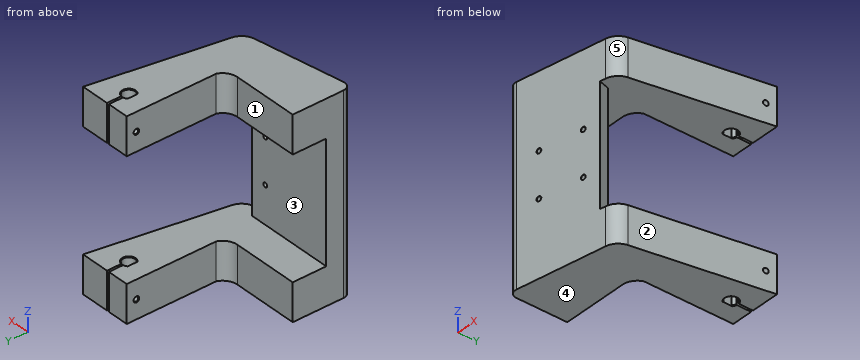
from build123d import *

# Parameters (mm, degrees)
BOSS_EXTRUDE1_DEPTH = 65
CUT_EXTRUDE1_DEPTH  = 40
CUT_EXTRUDE4_DEPTH  = 22.5
SKETCH11_W          = 20
SKETCH11_H          = 25
BOSS_EXTRUDE2_DEPTH = 10
BOSS_EXTRUDE6_DEPTH = 25
BOSS_EXTRUDE7_DEPTH = 25
CUT_EXTRUDE16_DEPTH = 130
SKETCH27_R          = 1.5
CUT_EXTRUDE17_DEPTH = 50
SKETCH28_R          = 1.7
CUT_EXTRUDE18_DEPTH = 50
BOSS_EXTRUDE8_DEPTH = 25
BOSS_EXTRUDE9_DEPTH = 25
CHAMFER9_SIZE       = 0.4
SKETCH31_R          = 1.5
CUT_EXTRUDE19_DEPTH = 10
FILLET1_R           = 0.2


with BuildPart() as part:
    # Sketch1 → Boss-Extrude1 (new body, symmetric)
    with BuildSketch(Plane.XY):
        with BuildLine():
            Line((0, 0), (0, -25.554938316))
            ThreePointArc((0, -25.554938316), (-2.359933303, -32.007021768), (-8.325876175, -35.413807897))
            Line((-8.325876175, -35.413807897), (-67.775097409, -45.508814922))
            ThreePointArc((-67.775097409, -45.508814922), (-71.838201048, -44.399413479), (-73.612159322, -40.579380131))
            Line((-73.612159322, -40.579380131), (-73.612159322, -6.5))
            Line((-73.612159322, -6.5), (-29.367881905, -6.5))
            ThreePointArc((-29.367881905, -6.5), (-23.632117541, -4.691520443), (-19.970955697, 0.079798567))
            Line((-19.970955697, 0.079798567), (-20, 0))
            Line((-20, 0), (0, 0))
        make_face()
    extrude(amount=BOSS_EXTRUDE1_DEPTH, both=True)

    # Sketch2 → Cut-Extrude1 (cut, symmetric)
    with BuildSketch(Plane.XY):
        with BuildLine():
            Line((-20, 0), (-19.970955697, 0.079798567))
            ThreePointArc((-19.970955697, 0.079798567), (-20.672372291, -1.438432196), (-21.617003148, -2.818534521))
            Line((-21.617003148, -2.818534521), (-12.102051753, -36.055036129))
            Line((-12.102051753, -36.055036129), (-8.325876175, -35.413807897))
            ThreePointArc((-8.325876175, -35.413807897), (-2.359933303, -32.007021768), (0, -25.554938316))
            Line((0, -25.554938316), (0, 0))
            Line((0, 0), (-20, 0))
        make_face()
    extrude(amount=CUT_EXTRUDE1_DEPTH, both=True, mode=Mode.SUBTRACT)

    # Sketch5 → Cut-Extrude4 (cut, symmetric)
    with BuildSketch(Plane(origin=(0, -6.5, 0), x_dir=(1, 0, 0), z_dir=(0, 1, 0))):
        Polygon((-73.612159322, 40), (-29.401702386, 40), (0, 40), (0, -40), (-29.367881905, -40), (-73.612159322, -40), align=None)
    extrude(amount=CUT_EXTRUDE4_DEPTH, both=True, mode=Mode.SUBTRACT)

    # Sketch11 → Boss-Extrude2 (add)
    with BuildSketch(Plane(origin=(0, 0, 0), x_dir=(1, 0, 0), z_dir=(0, 1, 0))):
        with Locations((-10, 52.5)):
            Rectangle(SKETCH11_W, SKETCH11_H)
        with Locations((-10, -52.5)):
            Rectangle(SKETCH11_W, SKETCH11_H)
    extrude(amount=BOSS_EXTRUDE2_DEPTH)

    # Sketch24 → Boss-Extrude6 (add)
    with BuildSketch(Plane(origin=(0, 0, -65), x_dir=(-1, 0, 0), z_dir=(0, 0, -1))):
        Polygon((0.147326036, -27.265147592), (-15, 60), (20, 60), (20, 0.001030349), align=None)
    extrude(amount=-BOSS_EXTRUDE6_DEPTH)

    # Sketch25 → Boss-Extrude7 (add)
    with BuildSketch(Plane.XY.offset(65)):
        Polygon((-0.147326036, -27.265147592), (-20, 0.001030349), (-20, 60), (15, 60), align=None)
    extrude(amount=-BOSS_EXTRUDE7_DEPTH)

    # Sketch26 → Cut-Extrude16 (cut)
    with BuildSketch(Plane(origin=(0, 0, -65), x_dir=(-1, 0, 0), z_dir=(0, 0, -1))):
        with BuildLine():
            Line((4.180094607, 50.081666326), (4.180094607, 61.21751544))
            Line((4.180094607, 61.21751544), (5.680094607, 61.21751544))
            Line((5.680094607, 61.21751544), (5.680094607, 50.081666326))
            ThreePointArc((5.680094607, 50.081666326), (4.930094607, 41.85), (4.180094607, 50.081666326))
        make_face()
    extrude(amount=-CUT_EXTRUDE16_DEPTH, mode=Mode.SUBTRACT)

    # Sketch27 → Cut-Extrude17 (cut)
    with BuildSketch(Plane.ZY.offset(20)):
        with Locations((-52.5, 53.5)):
            Circle(SKETCH27_R)
        with Locations((52.5, 53.5)):
            Circle(SKETCH27_R)
    extrude(amount=-CUT_EXTRUDE17_DEPTH, mode=Mode.SUBTRACT)

    # Sketch28 → Cut-Extrude18 (cut)
    with BuildSketch(Plane.ZY.offset(4.180094607)):
        with Locations((52.5, 53.5)):
            Circle(SKETCH28_R)
        with Locations((-52.5, 53.5)):
            Circle(SKETCH28_R)
    extrude(amount=-CUT_EXTRUDE18_DEPTH, mode=Mode.SUBTRACT)

    # Sketch29 → Boss-Extrude8 (add)
    with BuildSketch(Plane.XY.offset(65)):
        with BuildLine():
            Line((-8.080094607, 43.298148783), (-8.080094607, 48.701851217))
            ThreePointArc((-8.080094607, 48.701851217), (-9.080094607, 46), (-8.080094607, 43.298148783))
        make_face()
    extrude(amount=-BOSS_EXTRUDE8_DEPTH)

    # Sketch30 → Boss-Extrude9 (add)
    with BuildSketch(Plane.XY.offset(-40)):
        with BuildLine():
            Line((-8.080094607, 48.701851217), (-8.080094607, 43.298148783))
            ThreePointArc((-8.080094607, 43.298148783), (-9.080094607, 46), (-8.080094607, 48.701851217))
        make_face()
    extrude(amount=-BOSS_EXTRUDE9_DEPTH)

    # Chamfer9
    chamfer9_edges = [part.edges().sort_by_distance(p)[0] for p in [
        (-6.998541472, 49.597780922, 40),
        (-6.998541472, 49.597780922, -40),
        (-1.332313684, 43.931553135, -65),
        (-6.998541472, 49.597780922, 65),
        (-20, 53.5, -54),
        (-20, 53.5, 51),
        (-4.180094607, 53.5, 50.8),
        (-4.180094607, 53.5, -54.2),
        (-1.332313684, 43.931553135, 65),
        (-1.332313684, 43.931553135, 40),
        (-1.332313684, 43.931553135, -40),
        (-6.998541472, 49.597780922, -65),
    ]]
    chamfer(chamfer9_edges, length=CHAMFER9_SIZE)

    # Sketch31 → Cut-Extrude19 (cut)
    with BuildSketch(Plane(origin=(5.611689276, -33.047085202, 0), x_dir=(0.985886958, 0.167412383, 0), z_dir=(0.167412383, -0.985886958, 0))):
        with Locations((-29.287203222, 15)):
            Circle(SKETCH31_R)
        with Locations((-29.287203222, -15)):
            Circle(SKETCH31_R)
        with Locations((-59.287203222, -15)):
            Circle(SKETCH31_R)
        with Locations((-59.287203222, 15)):
            Circle(SKETCH31_R)
    extrude(amount=-CUT_EXTRUDE19_DEPTH, mode=Mode.SUBTRACT)

    # Fillet1
    fillet1_edges = [part.edges().sort_by_distance(p)[0] for p in [
        (-54.317621601, -43.223615721, 15),
        (-54.317621601, -43.223615721, -15),
        (-24.741012857, -38.201244245, -15),
        (-24.741012857, -38.201244245, 15),
    ]]
    fillet(fillet1_edges, radius=FILLET1_R)


solid = part.part
Source: CAD feature listing. Evaluate the final solid. Frame: model axes, mm. Face numbers are marked on the shaded views. A direction names the side the tool comes from. Coordinates: 2 decimals unless noted, no trailing zeros. Loops run counter-clockwise (first coordinate to the right, second up) from the corner with the lowest first, then second, coordinate; pieces in that order, holes last. Notation, with made-up numbers: (69.5, 4) -> (85.5, 4) arc R31 cw to (85.5, 31) -> close; hole circle Ø8 at (-34.75, -9). An arc over 180 degrees is marked (long way). Answer in a Markdown table with one row per item. Add a question column.
Q1. Reachability of the marked faces 1 and 2 from +Z, -Z, +X, -X, +Y, -Y: full face, straight path, thin tool, end or side. Return the list, or none.
Q2. Ray query, line 1 along Z through (x, y) = (3.5, 53.5); line 2 along Z through (x, y) = (-24, -28); line 3 along Y through (x, z) = (-11, 52). Return the intervals inside material, ascending.
Q3. Section B-B on y = 46. Return the cut outline in (x, z), and give its area (3 significant figures).
Q4. Section C-C on z = -38. Return the cut outline in (x, y), and give its area (3 significant figures).
Q5. Section D-D on y = 23.5. Return the cut outline in (x, z), and give its area (3 significant figures).
Q6. Section A-A on x = 3.5. Return the cut outline in (y, z), and give its area (3 significant figures).
Q7. Pull-direction query (Z, two-part tool) for the marked faces 3, 4 and 5; classes: pulls with the +Z half, pulls with the -Z half, needs draft (parallel to the pull), parting line crosses it, or undercut.
Q8. Contact query for flat-ended pins moving along their axis: pin 1 Ø4 at (y, z) = (53.5, 52.5) entering from -X; pin 2 Ø1 at (x, z) = (-30, 30.5) entering from +Y; pin 3 Ø5 at (x, y) = (-4.93, 46) entering from +Z; pin 4 Ø5 at (x, z) = (-11.5, -17) entering from -Y. Output: stop coordinate, or through.
Computed values:
| question | item | result |
|---|---|---|
| 1 | face 1 | +Z, -Z, -X, +Y |
| 1 | face 2 | +Z, -Z, +X, -Y |
| 2 | line 1 | z = -65 to -54.2, -50.8 to -40, 40 to 50.8, 54.2 to 65 |
| 2 | line 2 | z = -65 to -40, 40 to 65 |
| 2 | line 3 | y = -35.87 to 52.09, 54.91 to 60 |
| 3 | outline | (-20, -65) -> (-8.08, -65) -> (-8.08, -40) -> (-20, -40) -> close; (-20, 40) -> (-8.08, 40) -> (-8.08, 65) -> (-20, 65) -> close; (-0.78, -64.6) -> (-0.38, -65) -> (12.57, -65) -> (12.57, -40) -> (-0.38, -40) -> (-0.78, -40.4) -> close; (-0.78, 40.4) -> (-0.38, 40) -> (12.57, 40) -> (12.57, 65) -> (-0.38, 65) -> (-0.78, 64.6) -> close |
| 3 | area | 1,260 mm^2 |
| 4 | outline | (-73.61, -40.58) arc R5 ccw to (-67.78, -45.51) -> (-12.1, -36.06) -> (-14.12, -29) -> (-73.61, -29) -> close |
| 4 | area | 740 mm^2 |
| 5 | outline | (-20, -65) -> (8.66, -65) -> (8.66, -40) -> (-20, -40) -> close; (-20, 40) -> (8.66, 40) -> (8.66, 65) -> (-20, 65) -> close |
| 5 | area | 1,430 mm^2 |
| 6 | outline | (-6.25, -65) -> (60, -65) -> (60, -40) -> (-6.25, -40) -> close; (-6.25, 40) -> (60, 40) -> (60, 65) -> (-6.25, 65) -> close; hole circle Ø3.4 at (53.5, -52.5); hole circle Ø3.4 at (53.5, 52.5) |
| 6 | area | 3,290 mm^2 |
| 7 | face 3 | undercut |
| 7 | face 4 | pulls with the -Z half |
| 7 | face 5 | needs draft |
| 8 | pin 1 | stops at x = -20 |
| 8 | pin 2 | stops at y = -29 |
| 8 | pin 3 | passes through |
| 8 | pin 4 | stops at y = -36.38 |
